```python
from build123d import *

# Parameters (mm, degrees)
SKETCH2_W           = 6.35
SKETCH2_H           = 4.318
BOSS_EXTRUDE1_DEPTH = 6.35
SKETCH3_R           = 0.889
BOSS_EXTRUDE2_DEPTH = 0.889
CUT_EXTRUDE1_START  = -0.508
CUT_EXTRUDE1_DEPTH  = 0.508
SKETCH8_R           = 0.2032
BOSS_EXTRUDE3_DEPTH = 4.7752


with BuildPart() as part:
    # Sketch2 → Boss-Extrude1 (new body)
    with BuildSketch(Plane.XY):
        with Locations((2.667, -1.143)):
            Rectangle(SKETCH2_W, SKETCH2_H)
    extrude(amount=BOSS_EXTRUDE1_DEPTH)

    # Sketch3 → Boss-Extrude2 (add)
    with BuildSketch(Plane(origin=(5.842, 0, 0), x_dir=(0, 0, -1), z_dir=(1, 0, 0))):
        with Locations(Location((-5.08, -0.254, 0), (0, 0, 180))):
            Circle(SKETCH3_R)
    extrude(amount=BOSS_EXTRUDE2_DEPTH)

    # Sketch4 → Cut-Extrude1 (cut)
    with BuildSketch(Plane(origin=(6.731, 0, 0), x_dir=(0, 0, -1), z_dir=(1, 0, 0)).offset(CUT_EXTRUDE1_START)):
        with BuildLine():
            Line((-4.297980983, -0.676808772), (-5.502808772, 0.528019017))
            ThreePointArc((-5.502808772, 0.528019017), (-5.708617928, 0.374617928), (-5.862019017, 0.168808772))
            Line((-5.862019017, 0.168808772), (-4.657191228, -1.036019017))
            ThreePointArc((-4.657191228, -1.036019017), (-4.451382072, -0.882617928), (-4.297980983, -0.676808772))
        make_face()
    extrude(amount=CUT_EXTRUDE1_DEPTH, mode=Mode.SUBTRACT)

    # Sketch8 → Boss-Extrude3 (add)
    with BuildSketch(Plane(origin=(0, 0, 0), x_dir=(-1, 0, 0), z_dir=(0, 0, -1))):
        with Locations(Location((0, -2.286, 0), (0, 0, 180))):
            Circle(SKETCH8_R)
        with Locations(Location((-5.08, -2.286, 0), (0, 0, 180))):
            Circle(SKETCH8_R)
        with Locations(Location((-2.54, 0.254, 0), (0, 0, 180))):
            Circle(SKETCH8_R)
    extrude(amount=BOSS_EXTRUDE3_DEPTH)


solid = part.part
```
Could you check a few things on this model? Use its own coordinates, in mm. A direction names the side the tool comes from. Round coordinates to 2 decimals unless told otherwise and drop trailing zeros. Order: outer loops, then holes, each group sorted by start corner. A loop starts at its lowest first (then second) coordinate and runs counter-clockwise, first axis right, second up. Notation, with made-up numbers: (-16, 3) -> (-12, 3) arc R31 cw to (-12, 41) -> close; hole circle Ø7 at (-21.5, 69.25). An arc over 180 degrees is marked (long way). One line per question, with ' | ' between items.
Q1. If we section it at A-A on x = 0: Write out the boundary of the cut face in (y, z).
Computed values:
outline: (-3.3, 0) -> (-2.49, 0) -> (-2.49, -4.78) -> (-2.08, -4.78) -> (-2.08, 0) -> (1.02, 0) -> (1.02, 6.35) -> (-3.3, 6.35) -> close
Q2. Which directions (+Z, -Z, +X, -X, +Y, -Y) give clear straight access to the entire face, cutting with the end or side of a thin tool? Please do faces 4 (the face through (3, -3.302, 3)), 5 (the face through (6.473, -0.425, 5.268)).
Computed values:
face 4: +Z, -Z, +X, -X, -Y | face 5: +X
Q3. If I drill on line 1 (X direction, y = -0.9, z = 2); line 2 (Z direction, x = 0.5, y = -0.85); line 3 (Y direction, x = 5, z = -3), over which ranges is the centre line in solid material (lowest first)? Write a range as from..to.
Computed values:
line 1: -0.51..5.84 | line 2: 0..6.35 | line 3: -2.47..-2.1
Q4. If we section it at D-D on z = -2: Write out the boundary of the cut face in (x, y), plus the area to 3 significant figures.
Computed values:
outline: circle Ø0.41 at (0, -2.29); circle Ø0.41 at (2.54, 0.25); circle Ø0.41 at (5.08, -2.29) | area: 0.389 mm²
Q5. We'd pull the mould along Z, two halves only. Please class faces 1 (the face through (-0.508, -1, 3)), 2 (the face through (6.473, -0.083, 4.892)), 3 (the face through (3, -1, 0)): released by +Z, released by -Z, zero draft, split by the parting line, or undercut.
Computed values:
face 1: zero draft | face 2: undercut | face 3: released by -Z
Q6. If we section it at B-B on z = 5.08: Write out the boundary of the cut face in (x, y) (3 decimals), plus the area to 3 significant figures.
Computed values:
outline: (-0.508, -3.302) -> (5.842, -3.302) -> (5.842, -1.143) -> (6.731, -1.143) -> (6.731, -0.613) -> (6.223, -0.613) -> (6.223, 0.105) -> (6.731, 0.105) -> (6.731, 0.635) -> (5.842, 0.635) -> (5.842, 1.016) -> (-0.508, 1.016) -> close | area: 28.6 mm²
Q7. I'm going to push flat-ended pins straight in: pin 1 (1.3 mm diameter, centred on x = 1.5, y = -1.5, fed in from -Z); pin 2 (2 mm diameter, centred on x = 3.5, z = -2.5, fed in from +Y). Where does each tip first touch, or does it pass through?
Computed values:
pin 1: z = 0 | pin 2: y = 0.46
Q8. If we section it at C-C on y = -0.9: Write out the boundary of the cut face in (x, z), plus the area to 3 significant figures.
Computed values:
outline: (-0.51, 0) -> (5.84, 0) -> (5.84, 4.47) -> (6.22, 4.47) -> (6.22, 4.79) -> (6.73, 4.79) -> (6.73, 5.69) -> (5.84, 5.69) -> (5.84, 6.35) -> (-0.51, 6.35) -> close | area: 41.2 mm²
